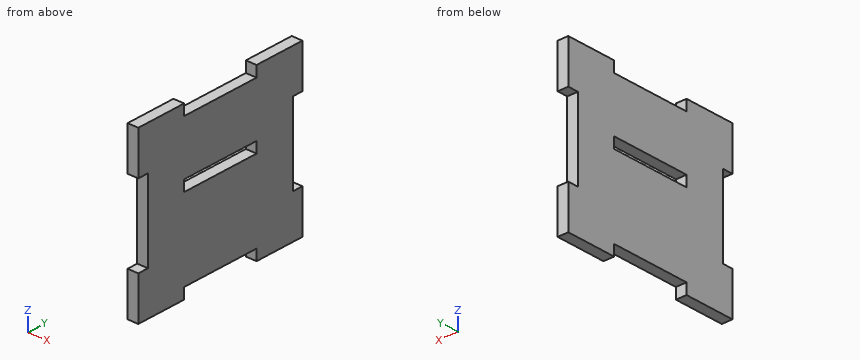
Autodesk Inventor part; units mm, degrees
ref_plane "YZ Plane" through (0, 0, 0) normal (1, 0, 0) x (0, 1, 0)
ref_plane "XZ Plane" through (0, 0, 0) normal (0, 1, 0) x (-1, 0, 0)
ref_plane "XY Plane" through (0, 0, 0) normal (0, 0, 1) x (1, 0, 0)
sketch "Skizze1" plane through (0, 0, 0) normal (1, 0, 0) x (0, 1, 0)
  line L0 (5.6933, -1.6012) -> (5.6933, -11.6012)
  line L1 (5.6933, -11.6012) -> (-69.3067, -11.6012)
  line L2 (-69.3067, -11.6012) -> (-69.3067, -1.6012)
  line L3 (-116.8067, -1.6012) -> (-69.3067, -1.6012)
  line L4 (5.6933, -1.6012) -> (53.1933, -1.6012)
  line L5 (5.6933, -156.6012) -> (5.6933, -146.6012)
  line L6 (5.6933, -146.6012) -> (-69.3067, -146.6012)
  line L7 (-69.3067, -146.6012) -> (-69.3067, -156.6012)
  line L8 (-69.3067, -61.6012) -> (5.6933, -61.6012)
  line L9 (5.6933, -61.6012) -> (5.6933, -71.6012)
  line L10 (5.6933, -71.6012) -> (-69.3067, -71.6012)
  line L11 (-69.3067, -71.6012) -> (-69.3067, -61.6012)
  line L12 (53.1933, -156.6012) -> (5.6933, -156.6012)
  line L13 (-69.3067, -156.6012) -> (-116.8067, -156.6012)
  line L14 (-116.8067, -41.6012) -> (-106.8067, -41.6012)
  line L15 (-106.8067, -41.6012) -> (-106.8067, -116.6012)
  line L16 (-106.8067, -116.6012) -> (-116.8067, -116.6012)
  line L17 (-116.8067, -156.6012) -> (-116.8067, -116.6012)
  line L18 (-116.8067, -41.6012) -> (-116.8067, -1.6012)
  line L19 (53.1933, -41.6012) -> (43.1933, -41.6012)
  line L20 (43.1933, -41.6012) -> (43.1933, -116.6012)
  line L21 (43.1933, -116.6012) -> (53.1933, -116.6012)
  line L22 (53.1933, -1.6012) -> (53.1933, -41.6012)
  line L23 (53.1933, -116.6012) -> (53.1933, -156.6012)
  point P0 (0, 0)
  dimension "d0" = 170
  dimension "d1" = 155
  dimension "d2" = 75
  dimension "d3" = 10
  dimension "d5" = 75
  dimension "d6" = 10
  dimension "d8" = 75
  dimension "d9" = 10
  dimension "d10" = 50
  dimension "d14" = 0
  dimension "d15" = 0
  dimension "d16" = 10
  dimension "d17" = 75
  dimension "d18" = 40
  dimension "d19" = 0
  dimension "d20" = 10
  dimension "d23" = 40
  dimension "d24" = 10
  dimension "d25" = 47.5
  dimension "d26" = 37.5
  dimension "d27" = 40
  dimension "d28" = 75
  dimension "d29" = 170
extrude "Extrusion1" add sketch "Skizze1" along normal blind 10
properties part number "Platte2-Seite"
Design review of the part built by this model. Coordinates are the model's own, in mm. Coordinates: 2 decimals unless noted, no trailing zeros. Loops run counter-clockwise (first coordinate to the right, second up) from the corner with the lowest first, then second, coordinate; pieces in that order, holes last.
Q1. For pin 1 (3 mm diameter, centred on x = 7, z = -96.5, fed in from -Y); pin 2 (5 mm diameter, centred on x = 5.5, z = -70.5, fed in from +Y), all flat-tipped, find the tip position at first contact; note any pin that passes through.
Reported:
pin 1: stops at y = -106.81
pin 2: stops at y = 43.19
Q2. We need section A-A on x = 6. State the section outline as (y, z) points, and give its area (3 significant figures).
Reported:
outline: (-116.81, -156.6) - (-69.31, -156.6) - (-69.31, -146.6) - (5.69, -146.6) - (5.69, -156.6) - (53.19, -156.6) - (53.19, -116.6) - (43.19, -116.6) - (43.19, -41.6) - (53.19, -41.6) - (53.19, -1.6) - (5.69, -1.6) - (5.69, -11.6) - (-69.31, -11.6) - (-69.31, -1.6) - (-116.81, -1.6) - (-116.81, -41.6) - (-106.81, -41.6) - (-106.81, -116.6) - (-116.81, -116.6) - close; hole (-69.31, -71.6) - (5.69, -71.6) - (5.69, -61.6) - (-69.31, -61.6) - close
area: 22,600 mm2
Q3. We need section B-B on y = -32.5. State the section outline as (x, z) points.
Reported:
outline: (0, -146.6) - (10, -146.6) - (10, -71.6) - (0, -71.6) - close; (0, -61.6) - (10, -61.6) - (10, -11.6) - (0, -11.6) - close
Q4. To check wall thickness, follow line 1 (Y direction, x = 3.5, z = -149); line 2 (Z direction, x = 1, y = -8.5); line 3 (Z direction, x = 5.25, y = -107). State the ranges of each line that lie inside material, in increasing order.
Reported:
line 1: y = -116.81 to -69.31, 5.69 to 53.19
line 2: z = -146.6 to -71.6, -61.6 to -11.6
line 3: z = -156.6 to -116.6, -41.6 to -1.6
